Input: part model. Units: mm. Frame: model coordinates. Face numbers are marked on the shaded views. Coordinates: 2 decimals unless noted, no trailing zeros. Order: outer loops, then holes, each group sorted by start corner. A loop starts at its lowest first (then second) coordinate and runs counter-clockwise, first axis right, second up. Notation, with made-up numbers: M 16.25,38.25 L 29.25,38.25 A5 ccw 29.25,47.25 Z; hole C -21.5,71.5 d4. An arc over 180 degrees is marked long. Answer in a Markdown table with one row per item.
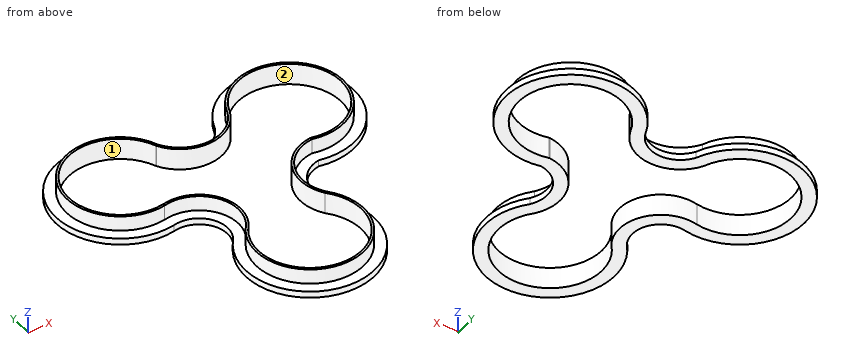
from build123d import *

# Parameters (mm, degrees)
F1_DEPTH = 3
F2_DEPTH = 10


with BuildPart() as f1:
    # F0 (on Top) → F1 (new body)
    with BuildSketch(Plane.XY):
        with BuildLine():
            ThreePointArc((11.75598, 34.46051), (-0.188241, 26.310271), (-12.897683, 33.206712))
            ThreePointArc((-12.897683, 33.206712), (-66.969323, 37.378844), (-35.915981, -7.082813))
            ThreePointArc((-35.915981, -7.082813), (-22.055212, -12.196979), (-21.628703, -26.964976))
            ThreePointArc((-21.628703, -26.964976), (0.871706, -76.686678), (23.722724, -27.12513))
            ThreePointArc((23.722724, -27.12513), (22.633328, -13.447379), (33.536886, -5.117908))
            ThreePointArc((33.536886, -5.117908), (66.226082, 38.654176), (11.75598, 34.46051))
        make_face()
        with BuildLine():
            ThreePointArc((-36.907983, -2.179073), (-62.499458, 35.120673), (-17.444433, 31.090865))
            ThreePointArc((-17.444433, 31.090865), (-0.055128, 21.310967), (16.39825, 32.594616))
            ThreePointArc((16.39825, 32.594616), (62.001748, 35.955299), (33.807071, -0.045165))
            ThreePointArc((33.807071, -0.045165), (18.206542, -11.104836), (19.741163, -30.166258))
            ThreePointArc((19.741163, -30.166258), (0.868135, -71.686626), (-17.640413, -30.002506))
            ThreePointArc((-17.640413, -30.002506), (-17.812054, -9.538309), (-36.907983, -2.179073))
        make_face(mode=Mode.SUBTRACT)
    extrude(amount=F1_DEPTH)

    # F0 (on Top) → F2 (join)
    with BuildSketch(Plane.XY):
        with BuildLine():
            ThreePointArc((16.39825, 32.594616), (-0.055128, 21.310967), (-17.444433, 31.090865))
            ThreePointArc((-17.444433, 31.090865), (-62.499458, 35.120673), (-36.907983, -2.179073))
            ThreePointArc((-36.907983, -2.179073), (-17.812054, -9.538309), (-17.640413, -30.002506))
            ThreePointArc((-17.640413, -30.002506), (0.868135, -71.686626), (19.741163, -30.166258))
            ThreePointArc((19.741163, -30.166258), (18.206542, -11.104836), (33.807071, -0.045165))
            ThreePointArc((33.807071, -0.045165), (62.001748, 35.955299), (16.39825, 32.594616))
        make_face()
        with BuildLine():
            ThreePointArc((-37.101393, -1.197366), (-61.627895, 34.630095), (-18.383489, 30.747101))
            Line((-18.383489, 30.747101), (-18.321174, 30.609903))
            ThreePointArc((-18.321174, 30.609903), (-0.010738, 20.311953), (17.314193, 32.193309))
            Line((17.314193, 32.193309), (17.340047, 32.258435))
            ThreePointArc((17.340047, 32.258435), (61.119406, 35.484691), (34.052515, 0.924246))
            Line((34.052515, 0.924246), (33.70776, 0.949892))
            ThreePointArc((33.70776, 0.949892), (17.300467, -10.681719), (18.914449, -30.728881))
            Line((18.914449, -30.728881), (18.990622, -30.827082))
            ThreePointArc((18.990622, -30.827082), (0.872515, -70.686635), (-16.895691, -30.669881))
            Line((-16.895691, -30.669881), (-16.808859, -30.55795))
            ThreePointArc((-16.808859, -30.55795), (-16.979997, -8.983359), (-37.101393, -1.197366))
        make_face(mode=Mode.SUBTRACT)
    extrude(amount=F2_DEPTH)


solid = f1.part
1) Cut plane A-A, the plane y = -19.5. Output: boundary loops of the cut face in (x, z).
Resolved:
| item | result |
|---|---|
| outline | M -19.58,0 L -13.58,0 L -13.58,10 L -14.58,10 L -14.58,3 L -19.58,3 Z; M 15.39,0 L 21.39,0 L 21.39,3 L 16.39,3 L 16.39,10 L 15.39,10 Z |
2) Contact query for flat-ended pins moving along their axis: pin 1 (12 mm diameter, centred on x = -30.5, y = -56.5, fed in from +Z); pin 2 (5 mm diameter, centred on x = -54, z = 6, fed in from -Y); pin 3 (1 mm diameter, centred on x = 13, z = 2.5, fed in from +Y). Output: stop coordinate, or through.
Resolved:
| item | result |
|---|---|
| pin 1 | stops at z = 3 |
| pin 2 | stops at y = -0.15 |
| pin 3 | stops at y = 38.36 |
3) Cut plane C-C, the plane x = -2.5. Output: boundary loops of the cut face in (y, z).
Resolved:
| item | result |
|---|---|
| outline | M -76.48,0 L -70.43,0 L -70.43,10 L -71.44,10 L -71.44,3 L -76.48,3 Z; M 20.36,0 L 26.39,0 L 26.39,3 L 21.36,3 L 21.36,10 L 20.36,10 Z |
4) Material intervals for probe 1 along X at (y, z) = (44.5, 2.25); probe 2 along X at (y, z) = (43.5, 1.25); probe 3 along Y at (x, z) = (9.5, 7.5), sorted ascending.
Resolved:
| item | result |
|---|---|
| probe 1 | x = -61.31 to -50.51, -31.34 to -20.53, 17.86 to 27.16, 52.73 to 62.02 |
| probe 2 | x = -62.34 to -52.53, -29.31 to -19.5, 16.98 to 25.69, 54.2 to 62.9 |
| probe 3 | y = -70.19 to -69.12, 23.23 to 24.41 |
5) Cut plane B-B, the plane z = 6.5. Output: boundary loops of the cut face in (x, y).
Resolved:
| item | result |
|---|---|
| outline | M -36.91,-2.18 A18.19 cw -17.64,-30 A25 ccw long 19.74,-30.17 A19.34 cw 33.81,-0.05 A25 ccw long 16.4,32.59 A18.88 cw -17.44,31.09 A25 ccw long Z; hole M -37.1,-1.2 A19.19 cw -16.81,-30.56 L -16.9,-30.67 A24 ccw long 18.99,-30.83 L 18.91,-30.73 A20.34 cw 33.71,0.95 L 34.05,0.92 A24 ccw long 17.34,32.26 L 17.31,32.19 A19.88 cw -18.32,30.61 L -18.38,30.75 A24 ccw long Z |
6) Mould query, pull axis Y, two halves, no side actions, for the marked faces 1 and 2. Classes: +Y half, -Y half, draft (parallel to the pull), parting line (faces both ways), or undercut.
Resolved:
| item | result |
|---|---|
| face 1 | undercut |
| face 2 | undercut |
